Autodesk Inventor part; units mm, degrees
ref_plane "YZ Plane" through (0, 0, 0) normal (1, 0, 0) x (0, 1, 0)
ref_plane "XZ Plane" through (0, 0, 0) normal (0, 1, 0) x (-1, 0, 0)
ref_plane "XY Plane" through (0, 0, 0) normal (0, 0, 1) x (1, 0, 0)
sketch "Skizze1" plane through (0, 0, 0) normal (0, 0, 1) x (1, 0, 0)
  line L0 (0, 0) -> (16, 0) construction
  line L1 (0, -5.75) -> (16, -5.75)
  line L2 (16, 5.75) -> (0, 5.75)
  arc A0 (0, 5.75) -> (0, -5.75) centre (0, 0) ccw
  arc A1 (16, -5.75) -> (16, 5.75) centre (16, 0) ccw
  point P0 (8, 0)
  dimension "d0" = 16
  dimension "d1" = 11.5
extrude "Extrusion1" add sketch "Skizze1" along normal blind 5.3
hole "Bohrung1" at (0, 0, 0) at (16, 0, 0) direction (0, 0, 1) diameter 3.4 end through all countersink diameter 7.5 countersink angle 90
fillet "Rundung1" radius 2 4 edges at (-5.75, 0, 0) (8, -5.75, 0) (21.75, 0, 0) (8, 5.75, 0)
properties part number "Connector_TopPlate"
Check sheet for the modelled part. Datum: model origin and axes. Units: mm. Round coordinates to 2 decimals unless told otherwise and drop trailing zeros. Write each loop counter-clockwise with the first axis right and the second up, starting at its lowest first coordinate (ties: lowest second). Pieces come first, ordered by that corner, then holes. Notation, with made-up numbers: M 28.5,73 L 64.5,73 A21 ccw 64.5,77 Z; hole C 61.25,-33 d10. An arc over 180 degrees is marked long. Write item = value, one per line. Start each with the question number.
1. Section check B-B, the plane z = 5. Record the cut outline in (x, y), then the cut area to 3 significant figures.
2. Gauge pin test, flat ends, axial feed: pin 1 (3 mm diameter, centred on x = 9.5, y = 3, fed in from -Z); pin 2 (1.5 mm diameter, centred on x = 12.5, z = 0.5, fed in from -Y); pin 3 (3 mm diameter, centred on x = 0, y = 0, fed in from -Z); pin 4 (1 mm diameter, centred on y = -2.5, z = 3, fed in from +X). Record the tip position at first contact, or that the pin passes through.
3. Scan lines: line 1 (X direction, y = 0, z = 3.1); line 2 (X direction, y = 0.5, z = 3.85); line 3 (Y direction, x = 16, z = 4.1). Record each from-to range of solid material in increasing order. Write a range as [from, to].
4. Section check D-D, the plane z = 1. Record the cut outline in (x, y).
5. Section check C-C, the plane x = 5.25. Record the cut outline in (y, z).
6. Section check A-A, the plane y = 0. State how many separate pieces and enclosed holes the cut face has, then the cut area to 3 significant figures.
7. Release check for a two-part mould opening along Y. For faces 1 (the flat face through (8, 0, 0)), 2 (the flat face through (8, 5.75, 4)), 3 (the cylindrical face through (14.314, -0.221, 3.698)) record: pulls with the +Y half, pulls with the -Y half, needs draft (parallel to the pull), parting line crosses it, or undercut.
Results found:
q1.outline = M 0,-5.75 L 16,-5.75 A5.75 ccw 16,5.75 L 0,5.75 A5.75 ccw Z; hole C 0,0 d3.4; hole C 16,0 d3.4
q1.area = 270 mm^2
q2.pin_1 = 0
q2.pin_2 = -5.6
q2.pin_3 = through
q2.pin_4 = 21.39
q3.line_1 = [-5.75, -1.7], [1.7, 14.3], [17.7, 21.75]
q3.line_2 = [-5.73, -1.62], [1.62, 14.38], [17.62, 21.73]
q3.line_3 = [-5.75, -1.7], [1.7, 5.75]
q4.outline = M 0,-5.48 L 16,-5.48 A5.48 ccw 16,5.48 L 0,5.48 A5.48 ccw Z; hole C 0,0 d5.5; hole C 16,0 d5.5
q5.outline = M -5.75,2 A2 ccw -3.75,0 L 3.75,0 A2 ccw 5.75,2 L 5.75,5.3 L -5.75,5.3 Z
q6.separate_pieces = 3
q6.enclosed_holes = 0
q6.area = 99.6 mm^2
q7.face_1 = needs draft
q7.face_2 = pulls with the +Y half
q7.face_3 = undercut
